Check sheet for the drawn part. Datum: minimum x, y, z corner. Units: mm. Round coordinates to 2 decimals unless told otherwise and drop trailing zeros. Loops run counter-clockwise (first coordinate to the right, second up) from the corner with the lowest first, then second, coordinate; pieces in that order, holes last.
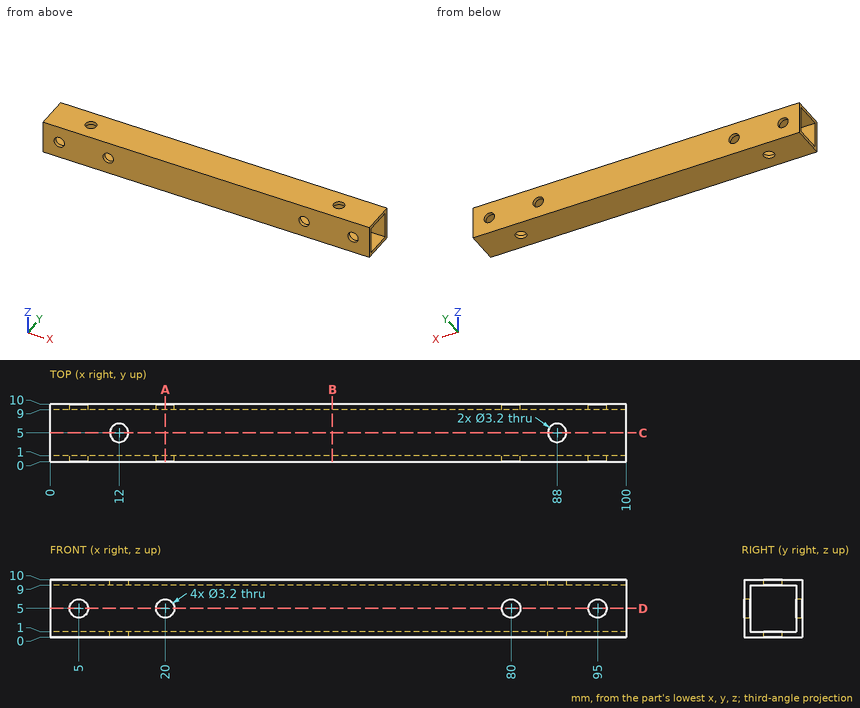
1. Gauge pin test, flat end, axial feed: P1, Ø3.5, axis at x = 88, y = 5, coming from the -Z side. Record the tip position at first contact, or that the pin passes through.
2. Section check A-A (x = 20). Enter the section's corners in (y, z).
3. Section check B-B (x = 49). Enter the section's corners in (y, z), then the cut area to 3 significant figures.
4. Section check D-D (z = 5). Give the number of separate pieces and of enclosed holes in the cut face, then the cut area to 3 significant figures.
5. Section check C-C (y = 5). Enter the section's corners in (x, z), then the cut area to 3 significant figures.
6. Scan lines: L1, parallel to X at y = 9.55, z = 5; L2, parallel to Y at x = 64.5, z = 3.75. Record each from-to range of solid material in increasing order.
Taken from the geometry:
1. P1: stops at z = 0
2. outline: (0, 0) - (10, 0) - (10, 3.4) - (9, 3.4) - (9, 1) - (1, 1) - (1, 3.4) - (0, 3.4) - close; (0, 6.6) - (1, 6.6) - (1, 9) - (9, 9) - (9, 6.6) - (10, 6.6) - (10, 10) - (0, 10) - close
3. outline: (0, 0) - (10, 0) - (10, 10) - (0, 10) - close; hole (1, 1) - (9, 1) - (9, 9) - (1, 9) - close
3. area: 36.0 mm2
4. separate pieces: 10
4. enclosed holes: 0
4. area: 174 mm2
5. outline: (0, 0) - (10.4, 0) - (10.4, 1) - (0, 1) - close; (0, 9) - (10.4, 9) - (10.4, 10) - (0, 10) - close; (13.6, 0) - (86.4, 0) - (86.4, 1) - (13.6, 1) - close; (13.6, 9) - (86.4, 9) - (86.4, 10) - (13.6, 10) - close; (89.6, 0) - (100, 0) - (100, 1) - (89.6, 1) - close; (89.6, 9) - (100, 9) - (100, 10) - (89.6, 10) - close
5. area: 187 mm2
6. L1: x = 0 to 3.4, 6.6 to 18.4, 21.6 to 78.4, 81.6 to 93.4, 96.6 to 100
6. L2: y = 0 to 1, 9 to 10
